```python
from build123d import *

# Parameters (mm, degrees)
SKETCH1_R           = 2
BOSS_EXTRUDE1_DEPTH = 6
SKETCH2_R           = 5.139196493
BOSS_EXTRUDE2_DEPTH = 6
SKETCH3_R           = 3.275
CUT_EXTRUDE1_DEPTH  = 10


with BuildPart() as part:
    # Sketch1 → Boss-Extrude1 (new body)
    with BuildSketch(Plane.XY):
        with BuildLine():
            ThreePointArc((12.495099897, 18.107249337), (10.42619144, 16.892644253), (8.810439427, 15.119231399))
            ThreePointArc((8.810439427, 15.119231399), (7.944379755, 15.591723167), (7.053068783, 16.014656467))
            ThreePointArc((7.053068783, 16.014656467), (7.538074714, 18.364213225), (7.304636989, 20.751922283))
            ThreePointArc((7.304636989, 20.751922283), (6.798373876, 20.923243358), (6.288098413, 21.082215689))
            ThreePointArc((6.288098413, 21.082215689), (4.695783155, 19.287729735), (3.707126384, 17.101819055))
            ThreePointArc((3.707126384, 17.101819055), (2.737446704, 17.283558272), (1.759066019, 17.410361505))
            ThreePointArc((1.759066019, 17.410361505), (1.494281102, 19.794797846), (0.534425957, 21.993507881))
            ThreePointArc((0.534425957, 21.993507881), (0, 22), (-0.534425957, 21.993507881))
            ThreePointArc((-0.534425957, 21.993507881), (-1.494281102, 19.794797846), (-1.759066019, 17.410361506))
            ThreePointArc((-1.759066019, 17.410361506), (-2.737446704, 17.283558272), (-3.707126384, 17.101819055))
            ThreePointArc((-3.707126384, 17.101819055), (-4.695783155, 19.287729736), (-6.288098413, 21.082215689))
            ThreePointArc((-6.288098413, 21.082215689), (-6.798373876, 20.923243359), (-7.30463699, 20.751922284))
            ThreePointArc((-7.30463699, 20.751922284), (-7.538074714, 18.364213226), (-7.053068783, 16.014656467))
            ThreePointArc((-7.053068783, 16.014656467), (-7.944379755, 15.591723167), (-8.810439427, 15.1192314))
            ThreePointArc((-8.810439427, 15.1192314), (-10.42619144, 16.892644253), (-12.495099898, 18.107249337))
            ThreePointArc((-12.495099898, 18.107249337), (-12.931275551, 17.798373876), (-13.35981926, 17.478993946))
            ThreePointArc((-13.35981926, 17.478993946), (-12.843989052, 15.136011463), (-11.656668033, 13.051325273))
            ThreePointArc((-11.656668033, 13.051325273), (-12.373661564, 12.373661564), (-13.051325273, 11.656668033))
            ThreePointArc((-13.051325273, 11.656668033), (-15.136011463, 12.843989052), (-17.478993946, 13.35981926))
            ThreePointArc((-17.478993946, 13.35981926), (-17.798373876, 12.931275551), (-18.107249337, 12.495099897))
            ThreePointArc((-18.107249337, 12.495099897), (-16.892644253, 10.42619144), (-15.1192314, 8.810439427))
            ThreePointArc((-15.1192314, 8.810439427), (-15.591723167, 7.944379755), (-16.014656467, 7.053068783))
            ThreePointArc((-16.014656467, 7.053068783), (-18.364213226, 7.538074714), (-20.751922283, 7.30463699))
            ThreePointArc((-20.751922283, 7.30463699), (-20.923243359, 6.798373876), (-21.082215689, 6.288098413))
            ThreePointArc((-21.082215689, 6.288098413), (-19.287729736, 4.695783155), (-17.101819055, 3.707126384))
            ThreePointArc((-17.101819055, 3.707126384), (-17.283558272, 2.737446704), (-17.410361505, 1.759066019))
            ThreePointArc((-17.410361505, 1.759066019), (-19.794797846, 1.494281102), (-21.993507881, 0.534425956))
            ThreePointArc((-21.993507881, 0.534425956), (-22, 0), (-21.993507881, -0.534425957))
            ThreePointArc((-21.993507881, -0.534425957), (-19.794797846, -1.494281102), (-17.410361505, -1.759066019))
            ThreePointArc((-17.410361505, -1.759066019), (-17.283558272, -2.737446704), (-17.101819055, -3.707126384))
            ThreePointArc((-17.101819055, -3.707126384), (-19.287729736, -4.695783155), (-21.082215689, -6.288098413))
            ThreePointArc((-21.082215689, -6.288098413), (-20.923243359, -6.798373876), (-20.751922283, -7.30463699))
            ThreePointArc((-20.751922283, -7.30463699), (-18.364213225, -7.538074714), (-16.014656467, -7.053068783))
            ThreePointArc((-16.014656467, -7.053068783), (-15.591723167, -7.944379755), (-15.1192314, -8.810439427))
            ThreePointArc((-15.1192314, -8.810439427), (-16.892644253, -10.42619144), (-18.107249337, -12.495099897))
            ThreePointArc((-18.107249337, -12.495099897), (-17.798373876, -12.93127555), (-17.478993946, -13.35981926))
            ThreePointArc((-17.478993946, -13.35981926), (-15.136011463, -12.843989052), (-13.051325272, -11.656668033))
            ThreePointArc((-13.051325272, -11.656668033), (-12.373661564, -12.373661564), (-11.656668033, -13.051325272))
            ThreePointArc((-11.656668033, -13.051325272), (-12.843989052, -15.136011463), (-13.35981926, -17.478993946))
            ThreePointArc((-13.35981926, -17.478993946), (-12.93127555, -17.798373876), (-12.495099897, -18.107249337))
            ThreePointArc((-12.495099897, -18.107249337), (-10.42619144, -16.892644253), (-8.810439427, -15.119231399))
            ThreePointArc((-8.810439427, -15.119231399), (-7.944379755, -15.591723167), (-7.053068783, -16.014656467))
            ThreePointArc((-7.053068783, -16.014656467), (-7.538074714, -18.364213225), (-7.304636989, -20.751922283))
            ThreePointArc((-7.304636989, -20.751922283), (-6.798373876, -20.923243358), (-6.288098413, -21.082215689))
            ThreePointArc((-6.288098413, -21.082215689), (-4.695783155, -19.287729735), (-3.707126384, -17.101819055))
            ThreePointArc((-3.707126384, -17.101819055), (-2.737446704, -17.283558272), (-1.759066019, -17.410361505))
            ThreePointArc((-1.759066019, -17.410361505), (-1.494281102, -19.794797846), (-0.534425956, -21.993507881))
            ThreePointArc((-0.534425956, -21.993507881), (0, -22), (0.534425957, -21.993507881))
            ThreePointArc((0.534425957, -21.993507881), (1.494281102, -19.794797846), (1.759066019, -17.410361505))
            ThreePointArc((1.759066019, -17.410361505), (2.737446704, -17.283558272), (3.707126384, -17.101819055))
            ThreePointArc((3.707126384, -17.101819055), (4.695783155, -19.287729735), (6.288098413, -21.082215689))
            ThreePointArc((6.288098413, -21.082215689), (6.798373876, -20.923243358), (7.304636989, -20.751922283))
            ThreePointArc((7.304636989, -20.751922283), (7.538074714, -18.364213225), (7.053068783, -16.014656467))
            ThreePointArc((7.053068783, -16.014656467), (7.944379755, -15.591723167), (8.810439427, -15.119231399))
            ThreePointArc((8.810439427, -15.119231399), (10.42619144, -16.892644253), (12.495099897, -18.107249337))
            ThreePointArc((12.495099897, -18.107249337), (12.93127555, -17.798373876), (13.359819259, -17.478993946))
            ThreePointArc((13.359819259, -17.478993946), (12.843989052, -15.136011463), (11.656668033, -13.051325272))
            ThreePointArc((11.656668033, -13.051325272), (12.373661564, -12.373661564), (13.051325272, -11.656668033))
            ThreePointArc((13.051325272, -11.656668033), (15.136011463, -12.843989052), (17.478993946, -13.35981926))
            ThreePointArc((17.478993946, -13.35981926), (17.798373876, -12.93127555), (18.107249337, -12.495099897))
            ThreePointArc((18.107249337, -12.495099897), (16.892644253, -10.42619144), (15.119231399, -8.810439427))
            ThreePointArc((15.119231399, -8.810439427), (15.591723167, -7.944379755), (16.014656467, -7.053068783))
            ThreePointArc((16.014656467, -7.053068783), (18.364213225, -7.538074714), (20.751922283, -7.304636989))
            ThreePointArc((20.751922283, -7.304636989), (20.923243358, -6.798373876), (21.082215689, -6.288098413))
            ThreePointArc((21.082215689, -6.288098413), (19.287729735, -4.695783155), (17.101819055, -3.707126384))
            ThreePointArc((17.101819055, -3.707126384), (17.283558272, -2.737446704), (17.410361505, -1.759066019))
            ThreePointArc((17.410361505, -1.759066019), (19.794797846, -1.494281102), (21.993507881, -0.534425956))
            ThreePointArc((21.993507881, -0.534425956), (22, 0), (21.993507881, 0.534425957))
            ThreePointArc((21.993507881, 0.534425957), (19.794797846, 1.494281102), (17.410361505, 1.759066019))
            ThreePointArc((17.410361505, 1.759066019), (17.283558272, 2.737446704), (17.101819055, 3.707126384))
            ThreePointArc((17.101819055, 3.707126384), (19.287729735, 4.695783155), (21.082215689, 6.288098413))
            ThreePointArc((21.082215689, 6.288098413), (20.923243358, 6.798373876), (20.751922283, 7.304636989))
            ThreePointArc((20.751922283, 7.304636989), (18.364213225, 7.538074714), (16.014656467, 7.053068783))
            ThreePointArc((16.014656467, 7.053068783), (15.591723167, 7.944379755), (15.119231399, 8.810439427))
            ThreePointArc((15.119231399, 8.810439427), (16.892644253, 10.42619144), (18.107249337, 12.495099897))
            ThreePointArc((18.107249337, 12.495099897), (17.798373876, 12.93127555), (17.478993946, 13.359819259))
            ThreePointArc((17.478993946, 13.359819259), (15.136011463, 12.843989052), (13.051325272, 11.656668033))
            ThreePointArc((13.051325272, 11.656668033), (12.373661564, 12.373661564), (11.656668033, 13.051325272))
            ThreePointArc((11.656668033, 13.051325272), (12.843989052, 15.136011463), (13.35981926, 17.478993946))
            ThreePointArc((13.35981926, 17.478993946), (12.93127555, 17.798373876), (12.495099897, 18.107249337))
        make_face()
        Circle(SKETCH1_R, mode=Mode.SUBTRACT)
    extrude(amount=BOSS_EXTRUDE1_DEPTH)

    # Sketch2 → Boss-Extrude2 (add)
    with BuildSketch(Plane.XY.offset(6)):
        Circle(SKETCH2_R)
    extrude(amount=-BOSS_EXTRUDE2_DEPTH)

    # Sketch3 → Cut-Extrude1 (cut)
    with BuildSketch(Plane.XY.offset(6)):
        Circle(SKETCH3_R)
    extrude(amount=-CUT_EXTRUDE1_DEPTH, mode=Mode.SUBTRACT)


solid = part.part
```
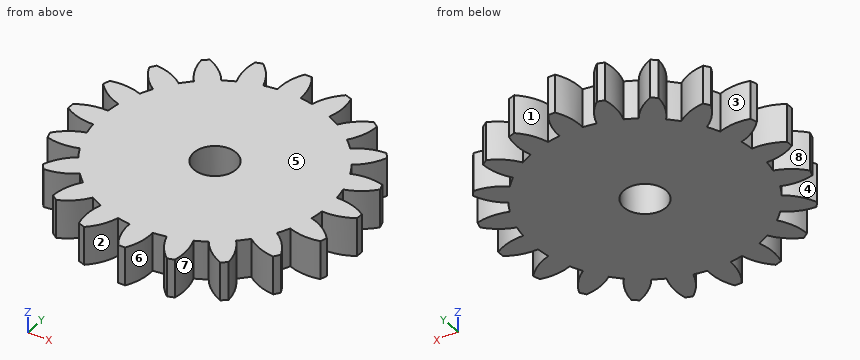
Geometry: final body of the model. Coordinates: model frame, mm. Face numbers are marked on the shaded views. A direction names the side the tool comes from. Round coordinates to 2 decimals unless told otherwise and drop trailing zeros. Write each loop counter-clockwise with the first axis right and the second up, starting at its lowest first coordinate (ties: lowest second). Pieces come first, ordered by that corner, then holes. Notation, with made-up numbers: (46, 70) -> (92, 70) arc R16 cw to (92, 89) -> close; hole circle Ø3 at (39.5, -20). An arc over 180 degrees is marked (long way). Return JSON: item names as keys, results as strings.
Q1. Set-up query: the marked faces 1, 2, 3 and 4. Return all of +Z, -Z, +X, -X, +Y, -Y with unobstructed straight access to the full face (end or side cutting, diameter ignored); none if empty.
From the geometry:
{"face 1": "+Z, -Z, +Y", "face 2": "+Z, -Z, -Y", "face 3": "+Z, -Z", "face 4": "+Z, -Z, -X"}
Q2. Section C-C on x = 5. Return the cut outline in (y, z).
From the geometry:
{"outline": "(-19.72, 0) -> (19.72, 0) -> (19.72, 6) -> (-19.72, 6) -> close"}
Q3. Mould query, pull axis X, two halves, no side actions, for the marked faces 5, 6, 7 and 8. Classes: +X half, -X half, draft (parallel to the pull), parting line (faces both ways), or undercut.
From the geometry:
{"face 5": "draft", "face 6": "undercut", "face 7": "undercut", "face 8": "-X half"}
Q4. Ray query, line 1 (X direction, y = -18, z = 5.2); line 2 (Y direction, x = 0, z = 1.6) (3 decimals); line 3 (X direction, y = -20, z = 2.4). Return the intervals inside material, ascending.
From the geometry:
{"line 1": "-12.65 to -12.24, -7.51 to -4.02, -1.76 to 1.76, 4.02 to 7.51, 12.24 to 12.65", "line 2": "-22 to -3.275, 3.275 to 22", "line 3": "-7.46 to -5.22, -1.44 to 1.44, 5.22 to 7.46"}
Q5. Section B-B on y = 9.5. Return the cut outline in (x, z).
From the geometry:
{"outline": "(-16.01, 0) -> (16.01, 0) -> (16.01, 6) -> (-16.01, 6) -> close"}
Q6. Section A-A on x = 0. Return the cut outline in (y, z) (3 decimals), and give its area (3 significant figures).
From the geometry:
{"outline": "(-22, 0) -> (-3.275, 0) -> (-3.275, 6) -> (-22, 6) -> close; (3.275, 0) -> (22, 0) -> (22, 6) -> (3.275, 6) -> close", "area": "225 mm2"}
Q7. First-contact query: pin 1 Ø1 at (y, z) = (-3.5, 3) entering from -X; pin 2 Ø5 at (x, y) = (-11.5, -2.5) entering from -Z; pin 3 Ø3 at (y, z) = (-5.5, 1) entering from +X; pin 4 Ø1 at (x, z) = (17.5, 4.5) entering from -Y. Flat tips, straight axial feed; report the tip coordinate or a pass-through.
From the geometry:
{"pin 1": "x = -17.96", "pin 2": "z = 0", "pin 3": "x = 21.08", "pin 4": "y = -13.36"}
